Autodesk Inventor part; units mm, degrees
ref_plane "YZ Plane" through (0, 0, 0) normal (1, 0, 0) x (0, 1, 0)
ref_plane "XZ Plane" through (0, 0, 0) normal (0, 1, 0) x (-1, 0, 0)
ref_plane "XY Plane" through (0, 0, 0) normal (0, 0, 1) x (1, 0, 0)
ref_plane "Work Plane1" through (0, 0, 0) normal (0, 0, 1) x (1, 0, 0)
ref_plane "Work Plane2" through (-27.9392, 13.2515, 3.3744) normal (0, 0, 1) x (1, 0.0042, 0)
sketch "Sketch4" plane through (-27.9392, 13.2515, 3.3744) normal (0, 0, 1) x (1, 0.0042, 0)
  circle A0 centre (0.0013, -0.0001) radius 12.5 construction
  line L0 (15.0013, 14.9999) -> (-14.9987, 14.9999) construction
  line L1 (-14.9987, 14.9999) -> (-14.9987, -40.0001) construction
  line L2 (-14.9987, -40.0001) -> (15.0013, -40.0001) construction
  line L3 (15.0013, -40.0001) -> (15.0013, 14.9999) construction
  line L4 (15.0013, 14.9999) -> (-14.9987, 14.9999)
  line L5 (-14.9987, 14.9999) -> (-14.9987, -40.0001)
  line L6 (-14.9987, -40.0001) -> (15.0013, -40.0001)
  line L7 (15.0013, -40.0001) -> (15.0013, 14.9999)
  circle A1 centre (0.0013, -0.0001) radius 10.3271
  circle A2 centre (-0.1451, -29.1987) radius 12.8 construction
  circle A3 centre (-0.1451, -29.6517) radius 8.1726 construction
  circle A4 centre (-0.1451, -29.6517) radius 8
  point P0 (27.8838, -13.3677)
  dimension "d13" = 15
  dimension "d14" = 15
  dimension "d15" = 15
  dimension "d16" = 40
  dimension "d17" = 16
  dimension "d34" = 29.652
extrude "Extrusion4" add sketch "Sketch4" along normal blind 2
sketch "Sketch5" plane through (-27.9392, 13.2515, 3.3744) normal (0, 0, -1) x (-1, -0.0042, 0)
  line L0 (15.2891, -0.4637) -> (15.1772, -1.9039) construction
  circle A0 centre (-0.0013, -0.0001) radius 12.5 construction
  line L1 (15.4424, -29.5809) -> (15.3809, -31.0242) construction
  circle A1 centre (-0.0013, -0.0001) radius 10.3271 construction
  circle A2 centre (0.1451, -29.6517) radius 8 construction
  line L2 (-15.0013, 14.9999) -> (14.9987, 14.9999) construction
  line L3 (-15.0013, -40.0001) -> (-15.0013, 14.9999) construction
  line L4 (14.9987, -40.0001) -> (-15.0013, -40.0001) construction
  line L5 (14.9987, 14.9999) -> (14.9987, -40.0001) construction
  line L6 (-15.0013, -40.0001) -> (14.7184, -40.0001)
  circle A3 centre (-0.0013, -0.0001) radius 15.2975 construction
  line L7 (14.9987, -40.0001) -> (-15.0013, -40.0001)
  line L8 (14.9987, 14.9999) -> (14.9987, -40.0001)
  line L9 (-15.0013, -40.0001) -> (-15.0013, 14.9999)
  line L10 (14.9987, 4.9557) -> (14.9987, 14.9999)
  arc A4 (5.5328, -14.7966) -> (14.9987, -4.956) centre (-0.0013, -0.0001) ccw
  line L11 (14.7184, -40.0001) -> (14.7184, -34.4839)
  line L12 (14.9987, -24.2596) -> (14.9987, -4.956)
  arc A5 (14.9987, -24.2596) -> (5.5328, -14.7966) centre (0.1451, -29.6517) ccw
  arc A6 (11.4871, -40.0001) -> (14.7184, -34.4839) centre (0.1451, -29.6517) ccw
  line L13 (-15.0013, 4.9557) -> (-15.0013, -4.956)
  line L14 (-15.0013, -33.4542) -> (-15.0013, -40.0001)
  arc A7 (-4.7152, -14.5532) -> (-15.0013, -24.943) centre (0.1451, -29.6517) ccw
  arc A8 (-15.0013, -33.4542) -> (-11.5503, -40.0001) centre (0.1451, -29.6517) ccw
  arc A9 (-15.0013, -4.956) -> (-5.4746, -14.8192) centre (-0.0013, -0.0001) ccw
  arc A10 (14.9987, 4.9557) -> (4.9545, 14.9999) centre (-0.0013, -0.0001) ccw
  arc A11 (-4.9572, 14.9999) -> (-15.0013, 4.9557) centre (-0.0013, -0.0001) ccw
  line L15 (14.9987, 14.9999) -> (3.0009, 14.9999)
  line L16 (-3.0035, 14.9999) -> (-15.0013, 14.9999)
  line L17 (-15.0013, -4.956) -> (-15.0013, -24.943)
  line L18 (14.9987, -4.956) -> (14.9987, -24.2596)
  point P0 (-27.8838, -13.3677)
  point P1 (10.9564, -8.3909)
extrude "Extrusion5" add sketch "Sketch5" along normal blind 7
sketch "Sketch6" plane through (-27.9392, 13.2515, -3.6256) normal (0, 0, -1) x (-1, -0.0042, 0)
  line L0 (-15.0013, -40.0001) -> (-11.5503, -40.0001)
  arc A0 (-5.4746, -14.8192) -> (-15.0013, -24.943) centre (0.1451, -29.6517) ccw
  line L1 (-15.0013, -33.4542) -> (-15.0013, -40.0001)
  line L2 (-15.0013, -4.956) -> (-15.0013, -24.943)
  line L3 (14.7184, -40.0001) -> (14.7184, -34.4839)
  line L4 (11.4871, -40.0001) -> (14.7184, -40.0001)
  arc A1 (-15.0013, -33.4542) -> (-11.5503, -40.0001) centre (0.1451, -29.6517) ccw
  arc A2 (-4.9572, 14.9999) -> (-15.0013, 4.9557) centre (-0.0013, -0.0001) ccw
  line L5 (-4.9572, 14.9999) -> (-15.0013, 14.9999)
  line L6 (-15.0013, 14.9999) -> (-15.0013, 4.9557)
  arc A3 (11.4871, -40.0001) -> (14.7184, -34.4839) centre (0.1451, -29.6517) ccw
  arc A4 (-15.0013, -4.956) -> (-5.4746, -14.8192) centre (-0.0013, -0.0001) ccw
  line L7 (-12.0013, 11.9999) -> (11.9987, 11.9999) construction
  line L8 (11.9987, 11.9999) -> (11.9987, -12.0001) construction
  line L9 (11.9987, -12.0001) -> (-12.0013, -12.0001) construction
  line L10 (-12.0013, -12.0001) -> (-12.0013, 11.9999) construction
  line L11 (-12.0013, 11.9999) -> (11.9987, -12.0001) construction
  line L12 (11.9987, 11.9999) -> (-12.0013, -12.0001) construction
  dimension "d32" = 24
  dimension "d33" = 24
hole "Hole1" at (-39.9878, 25.2013, -3.6256) at (-39.8879, 1.2015, -3.6256) at (-15.8881, 1.3014, -3.6256) at (-15.988, 25.3012, -3.6256) direction (0, 0, 1) diameter 2 depth 24 tip angle 118
sketch "Sketch7" plane through (-27.9392, 13.2515, -3.6256) normal (0, 0, -1) x (-1, -0.0042, 0)
  circle A0 centre (-0.0013, -0.0001) radius 10.3271
  line L0 (-12.0013, 11.9999) -> (11.9987, 11.9999) construction
  line L1 (11.9987, 11.9999) -> (11.9987, -12.0001) construction
  line L2 (11.9987, -12.0001) -> (-12.0013, -12.0001) construction
  line L3 (-12.0013, -12.0001) -> (-12.0013, 11.9999) construction
  line L4 (-12.0013, 11.9999) -> (11.9987, -12.0001) construction
  line L5 (11.9987, 11.9999) -> (-12.0013, -12.0001) construction
  point P0 (-27.8838, -13.3677)
  dimension "d30" = 24
  dimension "d31" = 24
properties part number "200_Gearbox_conterplate"
Geometry: final body of the model. Coordinates: model frame, mm. A direction names the side the tool comes from. Coordinates: 2 decimals unless noted, no trailing zeros. Order: outer loops, then holes, each group sorted by start corner. A loop starts at its lowest first (then second) coordinate and runs counter-clockwise, first axis right, second up.
(1) Section query D-D (y = 23). Return the cut outline in (x, z).
(2) Section query C-C (x = -24.5). Return the cut outline in (y, z).
(3) First-contact query: pin 1 (5 mm diameter, centred on x = -35.5, z = 4, fed in from -Y); pin 2 (3 mm diameter, centred on x = -16, z = 1.5, fed in from -Y); pin 3 (4 mm diameter, centred on x = -37.5, z = 2, fed in from +Y); pin 4 (13 mm diameter, centred on x = -27.96, y = -16.4, fed in from +Z). Flat tips, straight axial feed; report the tip coordinate or a pass-through.
(4) Draft query along X for faces 3 (the face through (-16.73, 1.84, 0.94)), 4 (the face through (-15, -2, -3.626)). Return one class per face: pulls with the +X half, pulls with the -X half, needs draft (parallel to the pull), parting line crosses it, or undercut.
(5) Section query A-A (x = -37.5). Return the cut outline in (y, z).
(6) Material intervals for probe 1 along X at (y, z) = (1.5, 5); probe 2 along X at (y, z) = (24.5, 3); probe 3 along Y at (x, z) = (-16.5, -3), sorted ascending.
(7) Access query for faces 1 (the face through (-41.198, -24.178, -0.077)), 2 (the face through (-34.33, -11.56, 4.36)). Directions: +Z, -Z, +X, -X, +Y, -Y. A direction counts if a zero-diameter tool reaches every point of the face in a straight line with its end or side. Return the directions, or none.
(8) Section query B-B (z = -1.25). State how many separate pieces and enclosed holes the cut face has, plus the area to 3 significant figures.
Solution:
1. outline: (-42.98, -3.63) - (-40.37, -3.63) - (-40.37, 3.37) - (-31.35, 3.37) - (-31.35, 5.37) - (-42.98, 5.37) - close; (-24.53, 3.37) - (-15.51, 3.37) - (-15.51, -3.63) - (-12.98, -3.63) - (-12.98, 5.37) - (-24.53, 5.37) - close
2. outline: (-26.73, 3.37) - (-23.61, 3.37) - (-23.61, 5.37) - (-26.73, 5.37) - close; (-9.19, 3.37) - (3.51, 3.37) - (3.51, 5.37) - (-9.19, 5.37) - close; (22.99, 3.37) - (28.27, 3.37) - (28.27, 5.37) - (22.99, 5.37) - close
3. pin 1: stops at y = -26.79
3. pin 2: stops at y = -26.7
3. pin 3: stops at y = 28.22
3. pin 4: passes through
4. face 3: undercut
4. face 4: needs draft
5. outline: (-26.79, 3.37) - (-3.8, 3.37) - (-3.8, -3.63) - (0.68, -3.63) - (0.68, 3.37) - (9.35, 3.37) - (9.35, 5.37) - (-26.79, 5.37) - close; (17.15, 3.37) - (25.83, 3.37) - (25.83, -3.63) - (28.21, -3.63) - (28.21, 5.37) - (17.15, 5.37) - close
6. probe 1: x = -42.89 to -40.84, -38.93 to -16.87, -14.91 to -12.89
6. probe 2: x = -42.99 to -40.7, -39.27 to -39.03, -16.85 to -16.59, -15.39 to -12.99
6. probe 3: y = -5.43 to 0.51, 2.09 to 2.35, 24.15 to 24.44, 26.16 to 28.3
7. face 1: -Z
7. face 2: +Z, -Z
8. separate pieces: 6
8. enclosed holes: 4
8. area: 202 mm2
